Check sheet for the modelled part. Datum: model origin and axes. Units: mm. Round coordinates to 2 decimals unless told otherwise and drop trailing zeros. Loops run counter-clockwise (first coordinate to the right, second up) from the corner with the lowest first, then second, coordinate; pieces in that order, holes last. Notation, with made-up numbers: (81, 29.5) -> (129, 29.5) arc R23 cw to (129, 66.5) -> close; hole circle Ø2 at (80, 83.5). An arc over 180 degrees is marked (long way). One line per question, with ' | ' between items.
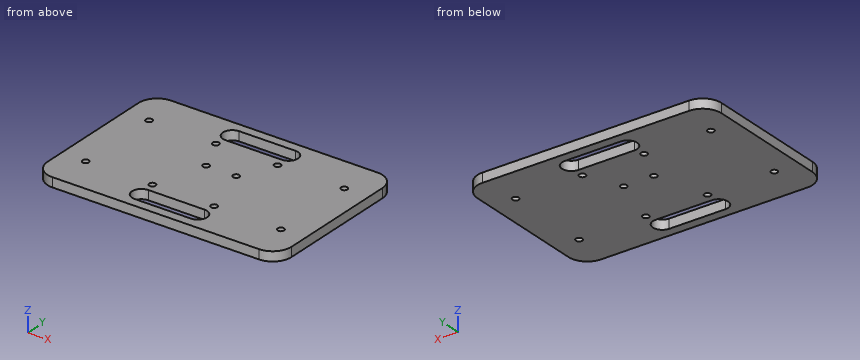
```python
from build123d import *

# Parameters (mm, degrees)
SKETCH1_R           = 1.7
BOSS_EXTRUDE1_DEPTH = 5


with BuildPart() as part:
    # Sketch1 → Boss-Extrude1 (new body)
    with BuildSketch(Plane.XY):
        with BuildLine():
            ThreePointArc((-55, 43), (-62.071067812, 40.071067812), (-65, 33))
            Line((-65, 33), (-65, -33))
            ThreePointArc((-65, -33), (-62.071067812, -40.071067812), (-55, -43))
            Line((-55, -43), (55, -43))
            ThreePointArc((55, -43), (62.071067812, -40.071067812), (65, -33))
            Line((65, -33), (65, 33))
            ThreePointArc((65, 33), (62.071067812, 40.071067812), (55, 43))
            Line((55, 43), (-55, 43))
        make_face()
        with Locations((52, -23)):
            Circle(SKETCH1_R, mode=Mode.SUBTRACT)
        with Locations((-52, -23)):
            Circle(SKETCH1_R, mode=Mode.SUBTRACT)
        with Locations((52, 23)):
            Circle(SKETCH1_R, mode=Mode.SUBTRACT)
        with Locations((-52, 23)):
            Circle(SKETCH1_R, mode=Mode.SUBTRACT)
        with BuildLine():
            ThreePointArc((15, 38), (20, 33), (15, 28))
            Line((15, 28), (-15, 28))
            ThreePointArc((-15, 28), (-20, 33), (-15, 38))
            Line((-15, 38), (15, 38))
        make_face(mode=Mode.SUBTRACT)
        with Locations((-16.44, -23)):
            Circle(SKETCH1_R, mode=Mode.SUBTRACT)
        with BuildLine():
            ThreePointArc((-15, -38), (-20, -33), (-15, -28))
            Line((-15, -28), (15, -28))
            ThreePointArc((15, -28), (20, -33), (15, -38))
            Line((15, -38), (-15, -38))
        make_face(mode=Mode.SUBTRACT)
        with Locations((16.44, -23)):
            Circle(SKETCH1_R, mode=Mode.SUBTRACT)
        with Locations((-8, 4.5)):
            Circle(SKETCH1_R, mode=Mode.SUBTRACT)
        with Locations((-16.44, 23)):
            Circle(SKETCH1_R, mode=Mode.SUBTRACT)
        with Locations((8, 4.5)):
            Circle(SKETCH1_R, mode=Mode.SUBTRACT)
        with Locations((16.44, 23)):
            Circle(SKETCH1_R, mode=Mode.SUBTRACT)
    extrude(amount=BOSS_EXTRUDE1_DEPTH)


solid = part.part
```
(1) Scan lines: probe 1 along Y at (x, z) = (52, 1.9); probe 2 along Y at (x, z) = (-12, 4.5); probe 3 along Y at (x, z) = (8, 2.9). Record each from-to range of solid material in increasing order.
Answer:
probe 1: y = -43 to -24.7, -21.3 to 21.3, 24.7 to 43 | probe 2: y = -43 to -38, -28 to 28, 38 to 43 | probe 3: y = -43 to -38, -28 to 2.8, 6.2 to 28, 38 to 43
(2) Sectioned sample at B-B, the plane y = 23. Record the cut outline in (x, z).
Answer:
outline: (-65, 0) -> (-53.7, 0) -> (-53.7, 5) -> (-65, 5) -> close; (-50.3, 0) -> (-18.14, 0) -> (-18.14, 5) -> (-50.3, 5) -> close; (-14.74, 0) -> (14.74, 0) -> (14.74, 5) -> (-14.74, 5) -> close; (18.14, 0) -> (50.3, 0) -> (50.3, 5) -> (18.14, 5) -> close; (53.7, 0) -> (65, 0) -> (65, 5) -> (53.7, 5) -> close
(3) Sectioned sample at D-D, the plane x = 52. Record the cut outline in (y, z).
Answer:
outline: (-43, 0) -> (-24.7, 0) -> (-24.7, 5) -> (-43, 5) -> close; (-21.3, 0) -> (21.3, 0) -> (21.3, 5) -> (-21.3, 5) -> close; (24.7, 0) -> (43, 0) -> (43, 5) -> (24.7, 5) -> close
(4) Sectioned sample at A-A, the plane x = -12. Record the cut outline in (y, z).
Answer:
outline: (-43, 0) -> (-38, 0) -> (-38, 5) -> (-43, 5) -> close; (-28, 0) -> (28, 0) -> (28, 5) -> (-28, 5) -> close; (38, 0) -> (43, 0) -> (43, 5) -> (38, 5) -> close
(5) Sectioned sample at C-C, the plane z = 2.5. Count the separate pieces of the cut face and the enclosed holes in it, and give its area (3 significant figures).
Answer:
separate pieces: 1 | enclosed holes: 12 | area: 10,200 mm2
